```python
from build123d import *

# Parameters (mm, degrees)
F0_W      = 126.9331611693
F0_H      = 100.463680923
F1_DEPTH  = 112.014
F2_R      = 12.7
F3_W      = 57.4507880956
F3_H      = 35.7939470559
F4_DEPTH  = 166.37
F5_DEPTH  = 99.822
F8_SIZE   = 7.62
F9_W      = 6.3165798783
F9_H      = 2.1055256948
F10_DEPTH = 148.844
F11_R     = 2.54


with BuildPart() as f1:
    # F0 (on Front) → F1 (new body)
    with BuildSketch(Plane.XZ):
        with Locations((3.1582918018, 3.759868443)):
            Rectangle(F0_W, F0_H)
    extrude(amount=F1_DEPTH)

    # F2
    f2_edges = [f1.edges().sort_by_distance(p)[0] for p in [
        (3.158292, -112.014, 53.991709),
        (66.624872, -56.007, 53.991709),
        (3.158292, 0, 53.991709),
        (-60.308289, -56.007, 53.991709),
    ]]
    fillet(f2_edges, radius=F2_R)


with BuildPart() as f4:
    # F3 (on Right) → F4 (new body)
    with BuildSketch(Plane.YZ):
        with Locations((-56.7088415846, -38.8018405065)):
            Rectangle(F3_W, F3_H)
    extrude(amount=F4_DEPTH)

    # F5 (add): a face of the model
    f5_faces = [f4.faces().sort_by_distance(p)[0] for p in [
        (166.37, -56.7088415846, -38.8018405065),
    ]]
    extrude(f5_faces, amount=F5_DEPTH)


with BuildPart() as f4_1:
    # F6: moved
    add(f4.part.moved(Location((-151.384, 0, 0))))


with BuildPart() as f1_1:
    add(f1.part)

    # F7: cut F4
    add(f4_1.part, mode=Mode.SUBTRACT)

    # F8
    f8_edges = [f1_1.edges().sort_by_distance(p)[0] for p in [
        (3.158292, -85.434236, -46.471972),
        (3.158292, -27.983448, -46.471972),
        (3.158292, -27.983448, -20.904867),
        (3.158292, -85.434236, -20.904867),
    ]]
    chamfer(f8_edges, length=F8_SIZE)

    # F9 (on Right) → F10 (cut)
    with BuildSketch(Plane.YZ):
        with Locations((-72.6506821811, -15.3402634896)):
            Rectangle(F9_W, F9_H)
    extrude(amount=F10_DEPTH, mode=Mode.SUBTRACT)

    # F11
    f11_edges = [f1_1.edges().sort_by_distance(p)[0] for p in [
        (66.624872, -56.708842, -20.904867),
    ]]
    fillet(f11_edges, radius=F11_R)


solid = f1_1.part
```
Read the model definition and answer for the solid it produces. Units are mm, in the model's axes. A direction names the side the tool comes from. Give positions to 0.01 mm unless a question says otherwise; leave off trailing zeros. Write each loop counter-clockwise with the first axis right and the second up, starting at its lowest first coordinate (ties: lowest second). Pieces come first, ordered by that corner, then holes. Notation, with made-up numbers: (70.25, -29) -> (123.25, -29) arc R11 cw to (123.25, -13) -> close; hole circle Ø2 at (43, 45). An arc over 180 degrees is marked (long way). Answer in a Markdown table with one row per item.
1) Section A-A on x = 43.5 is taken. Give the vertices of the cut face in (y, z), plus the area to 3 significant figures.
Results list:
| item | result |
|---|---|
| outline | (-112.01, -46.47) -> (-93.05, -46.47) -> (-85.43, -38.85) -> (-85.43, -28.52) -> (-77.81, -20.9) -> (-35.6, -20.9) -> (-27.98, -28.52) -> (-27.98, -38.85) -> (-20.36, -46.47) -> (0, -46.47) -> (0, 41.29) arc R12.7 ccw to (-12.7, 53.99) -> (-99.31, 53.99) arc R12.7 ccw to (-112.01, 41.29) -> close; hole (-75.81, -16.39) -> (-69.49, -16.39) -> (-69.49, -14.29) -> (-75.81, -14.29) -> close |
| area | 9,700 mm^2 |
2) Each of these flat-tipped pins is pushed along its axis until it touches: pin 1 Ø5 at (x, y) = (26.5, -25) entering from -Z; pin 2 Ø8 at (x, y) = (-8.5, -39) entering from -Z; pin 3 Ø7 at (x, y) = (18, -74) entering from -Z. Where does it stop, or does it pass through?
Results list:
| item | result |
|---|---|
| pin 1 | z = -44.34 |
| pin 2 | z = -21.51 |
| pin 3 | z = -20.9 |
3) A tool of negligible diameter and unlimited length cuts with its end or side. For faces 5 (the flat face through (2, -27.983, -34)), 6 (the cylindrical face through (63.003, -56.791, 50.173)), 7 (the flat face through (33, -73, -16.393)), from which of +Z, -Z, +X, -X, +Y, -Y can it reach the whole face along a straight path? Write none if from no direction.
Results list:
| item | result |
|---|---|
| face 5 | -Z, +X, -X |
| face 6 | +Z, +X, +Y, -Y |
| face 7 | +X |
4) Section D-D on x = -11 is taken. Give the vertices of the cut face in (y, z).
Results list:
| item | result |
|---|---|
| outline | (-112.01, -46.47) -> (-93.05, -46.47) -> (-85.43, -38.85) -> (-85.43, -28.52) -> (-77.81, -20.9) -> (-35.6, -20.9) -> (-27.98, -28.52) -> (-27.98, -38.85) -> (-20.36, -46.47) -> (0, -46.47) -> (0, 41.29) arc R12.7 ccw to (-12.7, 53.99) -> (-99.31, 53.99) arc R12.7 ccw to (-112.01, 41.29) -> close |
5) Section B-B on z = -23 is taken. Give the vertices of the cut face in (x, y), plus the area to 3 significant figures.
Results list:
| item | result |
|---|---|
| outline | (-60.31, -112.01) -> (66.62, -112.01) -> (66.62, -79.91) -> (-60.31, -79.91) -> close; (-60.31, -33.51) -> (66.62, -33.51) -> (66.62, 0) -> (-60.31, 0) -> close |
| area | 8,330 mm^2 |
6) Determine the mould class of faces 1 (the flat face through (2, 0, -2)), 2 (the flat face through (2, -55, 53.992)), 3 (the flat face through (2, -10, -46.472)), 4 (the flat face through (33, -73, -14.288)) for opening direction Z: released by +Z, released by -Z, zero draft, split by the parting line, or undercut.
Results list:
| item | result |
|---|---|
| face 1 | zero draft |
| face 2 | released by +Z |
| face 3 | released by -Z |
| face 4 | undercut |
7) Straight lines are drawn through the part: line 1 (Z direction, x = 49, y = -75); line 2 (Z direction, x = 22.5, y = -52.5); line 3 (Y direction, x = -5, z = -29.5). For each, find the intervals that lie inside material, in ascending order. Write a range as [from, to].
Results list:
| item | result |
|---|---|
| line 1 | [-20.9, -16.39], [-14.29, 53.99] |
| line 2 | [-20.9, 53.99] |
| line 3 | [-112.01, -85.43], [-27.98, 0] |
8) Section C-C on y = -59.5 is taken. Give the vertices of the cut face in (x, z), plus the area to 3 significant figures.
Results list:
| item | result |
|---|---|
| outline | (-60.31, -20.9) -> (64.08, -20.9) arc R2.54 ccw to (66.62, -18.36) -> (66.62, 41.29) arc R12.7 ccw to (53.92, 53.99) -> (-47.61, 53.99) arc R12.7 ccw to (-60.31, 41.29) -> close |
| area | 9,440 mm^2 |
